Source: CAD feature listing. Evaluate the final solid. Frame: model axes, mm. A direction names the side the tool comes from. Coordinates: 2 decimals unless noted, no trailing zeros. Order: outer loops, then holes, each group sorted by start corner. A loop starts at its lowest first (then second) coordinate and runs counter-clockwise, first axis right, second up.
```python
from build123d import *

# Parameters (mm, degrees)
ESQUISSE2_R             = 4.5
ESQUISSE2_R_2           = 5.375
ENL_V_MAT_EXTRU_1_DEPTH = 62.33292353
CHANFREIN2_SIZE         = 1


with BuildPart() as part:
    # Esquisse1 → Révolution1 (revolve)
    with BuildSketch(Plane.XY, mode=Mode.PRIVATE) as r_volution1_sk:
        with BuildLine():
            Line((-5.15, 0), (-30.25, 0))
            Line((-30.25, 0), (-22, 2.45))
            Line((-22, 2.45), (-5.15, 2.45))
            Line((-5.15, 2.45), (-5.15, 4))
            ThreePointArc((-5.15, 4), (-4.857106781, 4.707106781), (-4.15, 5))
            Line((-4.15, 5), (-3.196980896, 5))
            Line((-3.196980896, 5), (-2, 0))
            Line((-2, 0), (0, 0))
            Line((0, 0), (0, -41.5))
            Line((0, -41.5), (-0.522687484, -41.5))
            ThreePointArc((-0.522687484, -41.5), (-1.221634987, -41.215172978), (-1.522424218, -40.522944778))
            Line((-1.522424218, -40.522944778), (-2.197244162, -11.120075793))
            ThreePointArc((-2.197244162, -11.120075793), (-2.207114239, -11.001020564), (-2.231111264, -10.883991897))
            Line((-2.231111264, -10.883991897), (-5.15, 0))
        make_face()
    revolve(r_volution1_sk.sketch.rotate(Axis((0, 0, 0), (0, 1, 0)), 270), axis=Axis((0, 0, 0), (0, 1, 0)))

    # Esquisse2 → Enlèv. mat.-Extru.1 (cut, through all)
    with BuildSketch(Plane(origin=(0, 2.45, 0), x_dir=(1, 0, 0), z_dir=(0, 1, 0))):
        with Locations(Location((0, 16.55, 0), (0, 0, 270))):
            Circle(ESQUISSE2_R)
        with Locations(Location((-8.396893027, 8.396893027, 0), (0, 0, 270))):
            Circle(ESQUISSE2_R_2)
        with Locations(Location((8.396893027, 8.396893027, 0), (0, 0, 270))):
            Circle(ESQUISSE2_R_2)
        with Locations(Location((8.396893027, -8.396893027, 0), (0, 0, 270))):
            Circle(ESQUISSE2_R_2)
        with Locations(Location((0, -16.55, 0), (0, 0, 270))):
            Circle(ESQUISSE2_R)
        with Locations(Location((-8.396893027, -8.396893027, 0), (0, 0, 270))):
            Circle(ESQUISSE2_R_2)
    extrude(amount=-ENL_V_MAT_EXTRU_1_DEPTH, mode=Mode.SUBTRACT)

    # Chanfrein2
    chanfrein2_edges = [part.edges().sort_by_distance(p)[0] for p in [
        (-8.396893027, 2.45, -13.771893027),
        (8.396893027, 2.45, 3.021893027),
        (8.396893027, 2.45, -13.771893027),
        (-8.396893027, 2.45, 3.021893027),
    ]]
    chamfer(chanfrein2_edges, length=CHANFREIN2_SIZE)


solid = part.part
```
1. Pin query (flat end, axial travel): P1, Ø10, axis at x = 3, y = -10, coming from the +Z side; P2, Ø1, axis at x = -11.5, z = 14.5, coming from the +Y side; P3, Ø4, axis at x = -10.5, z = -16.5, coming from the -Y side. Return the tip coordinate at first contact, or that it passes through.
Findings:
P1: stops at z = 3.6
P2: stops at y = 2.45
P3: stops at y = 0
2. Access query for faces 4 (the face through (6.34, 0.74, -3.43)), 5 (the face through (5.028, 3.236, 1.116)), 6 (the face through (0.714, -25.616, -1.722)). Directions: +Z, -Z, +X, -X, +Y, -Y. A direction counts if a zero-diameter tool reaches every point of the face in a straight line with its end or side. Return the directions, or none.
Findings:
face 4: +Y, -Y
face 5: +Y
face 6: -Y
3. Section query B-B on y = -21. Return loops of the section in (x, z).
Findings:
outline: circle Ø3.94 at (0, 0)
4. Section query A-A on x = 7. Count the separate pieces of the cut face and the enclosed holes in it, plus the area to 3 significant figures.
Findings:
separate pieces: 3
enclosed holes: 0
area: 70.4 mm2
5. Ray query, line 1 (Y direction, x = 12.5, z = 3); line 2 (Y direction, x = -22.5, z = -8); line 3 (Z direction, x = -3, y = -7). Return the intervals inside material, ascending.
Findings:
line 1: y = 0 to 2.45
line 2: y = 0 to 1.89
line 3: z = -1.31 to 1.31
6. Draft query along Z for faces 1 (the face through (9, 2.45, 0)), 2 (the face through (-6.78, 0.74, -3.27)), 3 (the face through (13.63, 2.33, 17.78)). Return one class per face: released by +Z, released by -Z, zero draft, split by the parting line, or undercut.
Findings:
face 1: zero draft
face 2: undercut
face 3: split by the parting line
7. Section query C-C on y = -14. Return loops of the section in (x, z).
Findings:
outline: circle Ø4.26 at (0, 0)
